from build123d import *

# Parameters (mm, degrees)
SKETCH1_R           = 4.5
BOSS_EXTRUDE1_DEPTH = 16
SKETCH2_R           = 3.1
CUT_EXTRUDE1_DEPTH  = 3


with BuildPart() as part:
    # Sketch1 → Boss-Extrude1 (new body)
    with BuildSketch(Plane(origin=(0, 0, 0), x_dir=(1, 0, 0), z_dir=(0, 1, 0))):
        with Locations(Location((0, 0, 0), (0, 0, 270))):
            Circle(SKETCH1_R)
        with BuildLine():
            Line((1.506029548, 2.15), (-1.506029548, 2.15))
            ThreePointArc((-1.506029548, 2.15), (0, -2.625), (1.506029548, 2.15))
        make_face(mode=Mode.SUBTRACT)
    extrude(amount=BOSS_EXTRUDE1_DEPTH)

    # Sketch2 → Cut-Extrude1 (cut)
    with BuildSketch(Plane(origin=(0, 16, 0), x_dir=(1, 0, 0), z_dir=(0, 1, 0))):
        with Locations(Location((0, 0, 0), (0, 0, 270))):
            Circle(SKETCH2_R)
    extrude(amount=-CUT_EXTRUDE1_DEPTH, mode=Mode.SUBTRACT)


solid = part.part
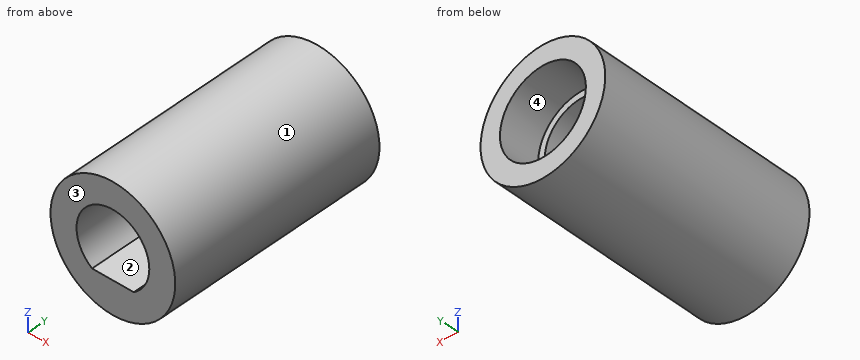
Can you work these out from the model? Positions are in its coordinate system, mm. Face numbers are marked on the shaded views. Give positions to 0.01 mm unless a question says otherwise; leave off trailing zeros. Loops run counter-clockwise (first coordinate to the right, second up) from the corner with the lowest first, then second, coordinate; pieces in that order, holes last. Notation, with made-up numbers: (77.25, -24.5) - (88.25, -24.5) arc R19 cw to (88.25, -2.5) - close; hole circle Ø8 at (26.5, 71.5). An arc over 180 degrees is marked (long way). Return JSON: item names as keys, results as strings.
1. I want a section at C-C on y = 10.75. Please give me the cut outline in (x, z) (3 decimals), and give its area (3 significant figures).
Output values:
{"outline": "circle Ø9 at (0, 0); hole (-1.506, -2.15) - (1.506, -2.15) arc R2.625 ccw (long way) to start", "area": "42.9 mm²"}
2. I want a section at B-B on x = 0. Please give me the cut outline in (y, z) (3 decimals), and give its area (3 significant figures).
Output values:
{"outline": "(0, -4.5) - (16, -4.5) - (16, -3.1) - (13, -3.1) - (13, -2.15) - (0, -2.15) - close; (0, 2.625) - (13, 2.625) - (13, 3.1) - (16, 3.1) - (16, 4.5) - (0, 4.5) - close", "area": "63.3 mm²"}
3. We'd pull the mould along Z, two halves only. Please class the marked faces 1, 2, 3 and 4: +Z half, -Z half, draft (parallel to the pull), parting line (faces both ways), or undercut.
Output values:
{"face 1": "parting line", "face 2": "undercut", "face 3": "draft", "face 4": "undercut"}
4. I want a section at D-D on z = -2.5. Please give me the cut outline in (x, y), and give its area (3 significant figures).
Output values:
{"outline": "(-3.74, 0) - (3.74, 0) - (3.74, 16) - (1.83, 16) - (1.83, 13) - (-1.83, 13) - (-1.83, 16) - (-3.74, 16) - close", "area": "109 mm²"}
5. I'm going to push flat-ended pins straight in: pin 1 Ø1.5 at (x, y) = (-2.5, 14) entering from -Z; pin 2 Ø1 at (y, z) = (13.5, 2.5) entering from -X; pin 3 Ø1 at (x, z) = (2, 0.5) entering from +Y. Where does each tip first touch, or does it pass through?
Output values:
{"pin 1": "stops at z = -4.15", "pin 2": "stops at x = -4.03", "pin 3": "passes through"}
6. I want a section at A-A on z = 0. Please give me the cut outline in (x, y) (3 decimals), and give its area (4 significant figures).
Output values:
{"outline": "(-4.5, 0) - (-2.625, 0) - (-2.625, 13) - (-3.1, 13) - (-3.1, 16) - (-4.5, 16) - close; (2.625, 0) - (4.5, 0) - (4.5, 16) - (3.1, 16) - (3.1, 13) - (2.625, 13) - close", "area": "57.15 mm²"}
7. If I drill on line 1 (X direction, y = 6.5, z = 0) (3 decimals); line 2 (Y direction, x = 2.25, z = -2); line 3 (X direction, y = 6.5, z = 1), over which ranges is the centre line in solid material (lowest first)?
Output values:
{"line 1": "x = -4.5 to -2.625, 2.625 to 4.5", "line 2": "y = 0 to 13", "line 3": "x = -4.39 to -2.43, 2.43 to 4.39"}
